```python
from build123d import *

# Parameters (mm, degrees)
SKETCH1_W           = 100
SKETCH1_H           = 90
BOSS_EXTRUDE2_DEPTH = 5
SKETCH2_R           = 6
SKETCH2_W           = 12
SKETCH2_H           = 11
SKETCH2_W_2         = 51
SKETCH2_H_2         = 20
SKETCH2_W_3         = 10
SKETCH2_H_3         = 8
SKETCH2_W_4         = 8
SKETCH2_H_4         = 6
CUT_EXTRUDE2_DEPTH  = 68.453687816


with BuildPart() as part:
    # Sketch1 → Boss-Extrude2 (new body)
    with BuildSketch(Plane(origin=(0, 0, 0), x_dir=(1, 0, 0), z_dir=(0, 1, 0))):
        Rectangle(SKETCH1_W, SKETCH1_H)
    extrude(amount=BOSS_EXTRUDE2_DEPTH)

    # Sketch2 → Cut-Extrude2 (cut, through all)
    with BuildSketch(Plane(origin=(0, 0, 0), x_dir=(1, 0, 0), z_dir=(0, 1, 0))):
        with Locations(Location((16.455886506, -25.155924864, 0), (0, 0, 270))):
            Circle(SKETCH2_R)
        with Locations((-32.037377006, 0.57672248)):
            Rectangle(SKETCH2_W, SKETCH2_H)
        with Locations((5.806889919, 24.732711273)):
            Rectangle(SKETCH2_W_2, SKETCH2_H_2)
        with Locations((-0.665141256, -29.560577811)):
            Rectangle(SKETCH2_W_3, SKETCH2_H_3)
        with Locations((-14.748919872, -30.448958229)):
            Rectangle(SKETCH2_W_4, SKETCH2_H_4)
    extrude(amount=CUT_EXTRUDE2_DEPTH, mode=Mode.SUBTRACT)


solid = part.part
```
Geometry: final body of the model. Coordinates: model frame, mm. A direction names the side the tool comes from. Coordinates: 2 decimals unless noted, no trailing zeros. Order: outer loops, then holes, each group sorted by start corner. A loop starts at its lowest first (then second) coordinate and runs counter-clockwise, first axis right, second up. Notation, with made-up numbers: M 51,79.5 L 86,79.5 A7 cw 86,92.5 Z; hole C -38,-28.5 d7. An arc over 180 degrees is marked long. Answer as CSV lines item,"result".
Q1. Section A-A on z = -29.5. Return the cut outline in (x, y).
Answers:
outline,"M -50,0 L -19.69,0 L -19.69,5 L -50,5 Z; M 31.31,0 L 50,0 L 50,5 L 31.31,5 Z"
Q2. Set-up query: faces 4 (the flat face through (-18.749, 2, 30)), 5 (the flat face through (-1, 2, -45)). Return all of +Z, -Z, +X, -X, +Y, -Y with unobstructed straight access to the full face (end or side cutting, diameter ignored); none if empty.
Answers:
face 4,"+Y, -Y"
face 5,"-Z, +X, -X, +Y, -Y"
Q3. Draft query along X for faces 1 (the flat face through (5, 2, -14.733)), 2 (the flat face through (-50, 2, 1)), 3 (the flat face through (-1, 5, -1)). Return one class per face: pulls with the +X half, pulls with the -X half, needs draft (parallel to the pull), parting line crosses it, or undercut.
Answers:
face 1,"undercut"
face 2,"pulls with the -X half"
face 3,"needs draft"
Q4. Section B-B on x = -29.5. Return the cut outline in (y, z), and give its area (3 significant figures).
Answers:
outline,"M 0,-45 L 5,-45 L 5,-6.08 L 0,-6.08 Z; M 0,4.92 L 5,4.92 L 5,45 L 0,45 Z"
area,"395 mm^2"
Q5. Section C-C on x = 18. Return the cut outline in (y, z).
Answers:
outline,"M 0,-45 L 5,-45 L 5,-34.73 L 0,-34.73 Z; M 0,-14.73 L 5,-14.73 L 5,19.36 L 0,19.36 Z; M 0,30.95 L 5,30.95 L 5,45 L 0,45 Z"
Q6. Section D-D on y = 2.4. Return the cut outline in (x, z), and give its area (3 significant figures).
Answers:
outline,"M -50,-45 L 50,-45 L 50,45 L -50,45 Z; hole M -38.04,-6.08 L -26.04,-6.08 L -26.04,4.92 L -38.04,4.92 Z; hole M -19.69,-34.73 L 31.31,-34.73 L 31.31,-14.73 L -19.69,-14.73 Z; hole M -18.75,27.45 L -10.75,27.45 L -10.75,33.45 L -18.75,33.45 Z; hole M -5.67,25.56 L 4.33,25.56 L 4.33,33.56 L -5.67,33.56 Z; hole C 16.46,25.16 d12"
area,"7,610 mm^2"
Q7. First-contact query: P1, Ø7, axis at x = 16.46, z = 25.16, coming from the +Y side. Flat tip, straight axial feed; report the tip coordinate or a pass-through.
Answers:
P1,"passes through"
Q8. Line query: probe 1 along Z at (x, y) = (-18.5, 4.2); probe 2 along X at (y, z) = (4, -27); probe 3 along Z at (x, y) = (3.5, 2.5). Output: solid intervals per line, ascending. Write a range as [from, to].
Answers:
probe 1,"z = [-45, -34.73], [-14.73, 27.45], [33.45, 45]"
probe 2,"x = [-50, -19.69], [31.31, 50]"
probe 3,"z = [-45, -34.73], [-14.73, 25.56], [33.56, 45]"
